Design review of the part built by this model. Coordinates are the model's own, in mm. Face numbers are marked on the shaded views. A direction names the side the tool comes from. Round coordinates to 2 decimals unless told otherwise and drop trailing zeros. Order: outer loops, then holes, each group sorted by start corner. A loop starts at its lowest first (then second) coordinate and runs counter-clockwise, first axis right, second up. Notation, with made-up numbers: (67, 61) - (97, 61) arc R26 cw to (97, 82) - close; hole circle Ø1 at (42.5, -2.75). An arc over 180 degrees is marked (long way). Answer as a JSON object with one key per item and string values. Group by question number.
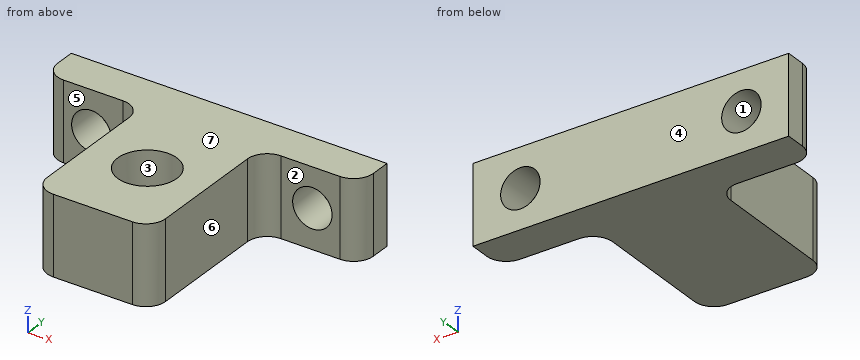
Solid Edge part; units mm, degrees
sketch "Sketch1" plane through (0, 0, 0) normal (0, 0, 1) x (1, 0, 0)
  line L0 (-25.4, 19.05) -> (25.4, 19.05)
  line L1 (25.4, 19.05) -> (25.4, 12.7)
  line L2 (25.4, 12.7) -> (9.525, 12.7)
  line L3 (9.525, 12.7) -> (9.525, -12.7)
  line L4 (9.525, -12.7) -> (-9.525, -12.7)
  line L5 (-9.525, -12.7) -> (-9.525, 12.7)
  line L6 (-9.525, 12.7) -> (-25.4, 12.7)
  line L7 (-25.4, 12.7) -> (-25.4, 19.05)
  dimension "D1" = 25.4
  dimension "D2" = 9.525
  dimension "D3" = 25.4
  dimension "D4" = 25.4
  dimension "D5" = 9.525
  dimension "D6" = 9.525
  dimension "D7" = 25.4
  dimension "D8" = 9.525
extrude "Protrusion1" add sketch "Sketch1" along normal blind 12.7
fillet "Round_1" radius 3.175 6 edges at (9.525, 12.7, 6.35) (9.525, -12.7, 6.35) (-9.525, -12.7, 6.35) (25.4, 12.7, 6.35) (-9.525, 12.7, 6.35) (-25.4, 12.7, 6.35)
sketch "Sketch2" plane through (0, 3.175, 12.7) normal (0, 0, 1) x (0, 1, 0)
  circle A0 centre (-3.175, 0) radius 4.7625
extrude "PivotHole" cut sketch "Sketch2" against normal blind 10.16
sketch "Sketch3" plane through (-17.4625, 12.7, 6.35) normal (0, -1, 0) x (1, 0, 0)
  circle A0 centre (-0.3175, 0) radius 3.175
  dimension "D1" = 0.3175
extrude "v_1" cut sketch "Sketch3" against normal blind 25.4
mirror "Mirror1" about plane through (0, 0, 0) normal (1, 0, 0) of "v_1"
properties material "Aluminum, 6061-T6"
1. To check wall thickness, follow line 1 (Z direction, x = -17.78, y = 17) (3 decimals); line 2 (X direction, y = 0, z = 7.75) (1 decimal); line 3 (X direction, y = 1.5, z = 2.5) (3 decimals). State the ranges of each line that lie inside material, in increasing order. Write a range as from..to.
2. Take a section at D-D, the plane y = 0. Give the boundary of the cut face in (x, z) (1 decimal), then the cut area to 3 significant figures.
3. Tool access review of the marked faces 5, 6 and 7: name each direction out of +Z, -Z, +X, -X, +Y, -Y from which nothing blocks a thin tool from reaching the whole face with its end or side.
4. Take a section at A-A, the plane z = 6.35. Count the separate pieces of the cut face and the enclosed holes in it, then the cut area to 3 significant figures.
5. Take a section at B-B, the plane x = -17.78. Give the boundary of the cut face in (y, z) (3 decimals).
6. Clearance check with flat-ended pins moving along their axes: P1, Ø2, axis at x = 12.5, z = 5.5, coming from the -Y side; P2, Ø1, axis at y = -2.5, z = 3.5, coming from the -X side (3 decimals); P3, Ø6.5, axis at y = 0.5, z = 4.5, coming from the +X side (3 decimals). State where each tip first meets the part, or that it passes through.
7. Mouldability with a two-part tool opening along Y and no side actions: class the marked faces 1, 2, 3 and 4 as pulls with the +Y half, pulls with the -Y half, needs draft (parallel to the pull), parting line crosses it, or undercut.
Response values:
{
 "1": {"line 1": "0..3.175, 9.525..12.7", "line 2": "-9.5..-4.8, 4.8..9.5", "line 3": "-9.525..9.525"},
 "2": {"outline": "(-9.5, 0) - (9.5, 0) - (9.5, 12.7) - (4.8, 12.7) - (4.8, 2.5) - (-4.8, 2.5) - (-4.8, 12.7) - (-9.5, 12.7) - close", "area": "145 mm2"},
 "3": {"face 5": "+Z, -Z, -X, -Y", "face 6": "+Z, -Z, +X, -Y", "face 7": "+Z, +X, -X, +Y, -Y"},
 "4": {"separate pieces": "3", "enclosed holes": "1", "area": "650 mm2"},
 "5": {"outline": "(12.7, 0) - (19.05, 0) - (19.05, 3.175) - (12.7, 3.175) - close; (12.7, 9.525) - (19.05, 9.525) - (19.05, 12.7) - (12.7, 12.7) - close"},
 "6": {"P1": "y = 12.46", "P2": "x = -9.525", "P3": "x = 9.525"},
 "7": {"face 1": "needs draft", "face 2": "pulls with the -Y half", "face 3": "undercut", "face 4": "pulls with the +Y half"}
}
